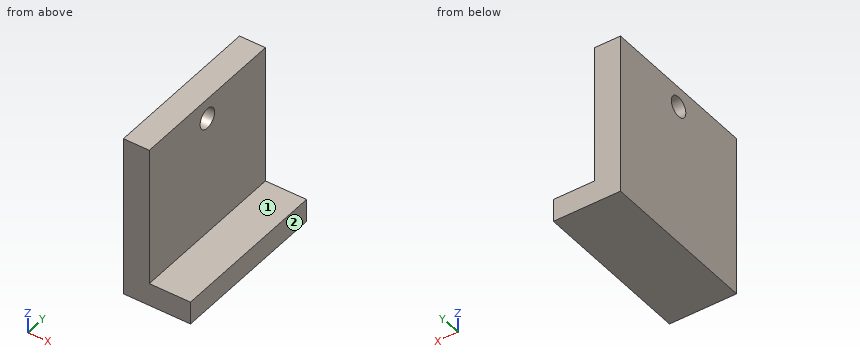
```python
from build123d import *

# Parameters (mm, degrees)
F0_W     = 25.4
F0_H     = 25.4
F1_DEPTH = 25.4
F2_W     = 7.143348
F2_H     = 25.4
F3_DEPTH = 25.4
F4_R     = 1.5875
F5_DEPTH = 25.4


with BuildPart() as f1:
    # F0 (on Front) → F1 (new body)
    with BuildSketch(Plane.XZ):
        with Locations((12.7, 12.7)):
            Rectangle(F0_W, F0_H)
    extrude(amount=F1_DEPTH)

    # F2 (on face) → F3 (cut)
    with BuildSketch(Plane.XZ.offset(25.4)):
        with Locations((3.571674, 12.7)):
            Rectangle(F2_W, F2_H)
        Polygon((25.4, 25.4), (11.18654, 25.4), (11.18654, 3.579036), (17.612327, 3.579036), (17.612327, 0), (25.4, 0), align=None)
    extrude(amount=-F3_DEPTH, mode=Mode.SUBTRACT)

    # F4 (on face) → F5 (cut)
    with BuildSketch(Plane(origin=(7.143348, 0, 0), x_dir=(0, -1, 0), z_dir=(-1, 0, 0))):
        with Locations((12.7, 22.225)):
            Circle(F4_R)
    extrude(amount=-F5_DEPTH, mode=Mode.SUBTRACT)


solid = f1.part
```
For this review, take the finished solid that the model builds, in its own axes (mm). Face numbers are marked on the shaded views. A direction names the side the tool comes from. Coordinates: 2 decimals unless noted, no trailing zeros. Loops run counter-clockwise (first coordinate to the right, second up) from the corner with the lowest first, then second, coordinate; pieces in that order, holes last.
1. Add section C-C, the plane x = 15. Give the boundary of the cut face in (y, z).
2. For the marked faces 1 and 2, list the 3-axis set-ups (+Z, -Z, +X, -X, +Y, -Y) from which the entire face can be reached by the end or side of a thin tool; tool diameter is ignored.
3. Add section D-D, the plane z = 7. Give the boundary of the cut face in (x, y).
4. Insertion check: P1, Ø1, axis at y = -14.5, z = 14, coming from the +X side. The pin has a flat end and moves straight along its axis. Give the tip position at first contact, or say it passes through.
5. Add section A-A, the plane y = -12.7. Give the boundary of the cut face in (x, z), then the cut area to 3 significant figures.
6. For line 1 (Z direction, x = 10.2, y = -12.7); line 2 (X direction, y = -16.25, z = 5); line 3 (Y direction, x = 9.5, z = 23.5), list the stretches that pass through material, from the lowest coordinate up.
7. Add section B-B, the plane y = -16.75. Give the boundary of the cut face in (x, z), then the cut area to 3 significant figures.
Result:
1. outline: (-25.4, 0) - (0, 0) - (0, 3.58) - (-25.4, 3.58) - close
2. face 1: +Z, +X, +Y, -Y
2. face 2: +Z, -Z, +X, +Y, -Y
3. outline: (7.14, -25.4) - (11.19, -25.4) - (11.19, 0) - (7.14, 0) - close
4. P1: stops at x = 11.19
5. outline: (7.14, 0) - (17.61, 0) - (17.61, 3.58) - (11.19, 3.58) - (11.19, 20.64) - (7.14, 20.64) - close; (7.14, 23.81) - (11.19, 23.81) - (11.19, 25.4) - (7.14, 25.4) - close
5. area: 113 mm2
6. line 1: z = 0 to 20.64, 23.81 to 25.4
6. line 2: x = 7.14 to 11.19
6. line 3: y = -25.4 to -13.65, -11.75 to 0
7. outline: (7.14, 0) - (17.61, 0) - (17.61, 3.58) - (11.19, 3.58) - (11.19, 25.4) - (7.14, 25.4) - close
7. area: 126 mm2
